Can you work these out from the drawing? Everything is in mm from the part's minimum corner. Coordinates: 2 decimals unless noted, no trailing zeros. Loops run counter-clockwise (first coordinate to the right, second up) from the corner with the lowest first, then second, coordinate; pieces in that order, holes last. Notation, with made-up numbers: (-14.5, 2.5) - (44.5, 2.5) arc R26 ccw to (44.5, 25.5) - close; hole circle Ø8 at (42, -11). An arc over 180 degrees is marked (long way). One line per question, with ' | ' between items. Start each with the question number.
1. I want a section at B-B, the plane y = 0.6. Count the separate pieces of the cut face and the enclosed holes in it, then the cut area to 3 significant figures.
2. I want a section at C-C, the plane z = 2.75. Write out the boundary of the cut face in (x, y).
3. I want a section at D-D, the plane x = 5.25. Write out the boundary of the cut face in (y, z), then the cut area to 3 significant figures.
4. We'd pull the mould along X, two halves only. Please class the marked faces 1, 2 and 3: pulls with the +X half, pulls with the -X half, needs draft (parallel to the pull), parting line crosses it, or undercut.
5. I'm going to push flat-ended pins straight in: P1, Ø1.3, axis at x = 7, y = 1.5, coming from the +Z side; P2, Ø1.3, axis at x = 10.5, y = 1, coming from the +Z side; P3, Ø0.6, axis at x = 7.5, y = 1, coming from the -Z side; P4, Ø4, axis at x = 14, z = 9.16, coming from the +Y side. Where does each tip first touch, or does it pass through?
6. I want a section at A-A, the plane x = 9. Write out the boundary of the cut face in (y, z).
7. Please list where these lines run through material, in increasing order: L1, parallel to X at y = 1, z = 9; L2, parallel to X at y = 1.55, z = 10.25; L3, parallel to X at y = 1.45, z = 11.25 (1 decimal). Write a range as [from, to].
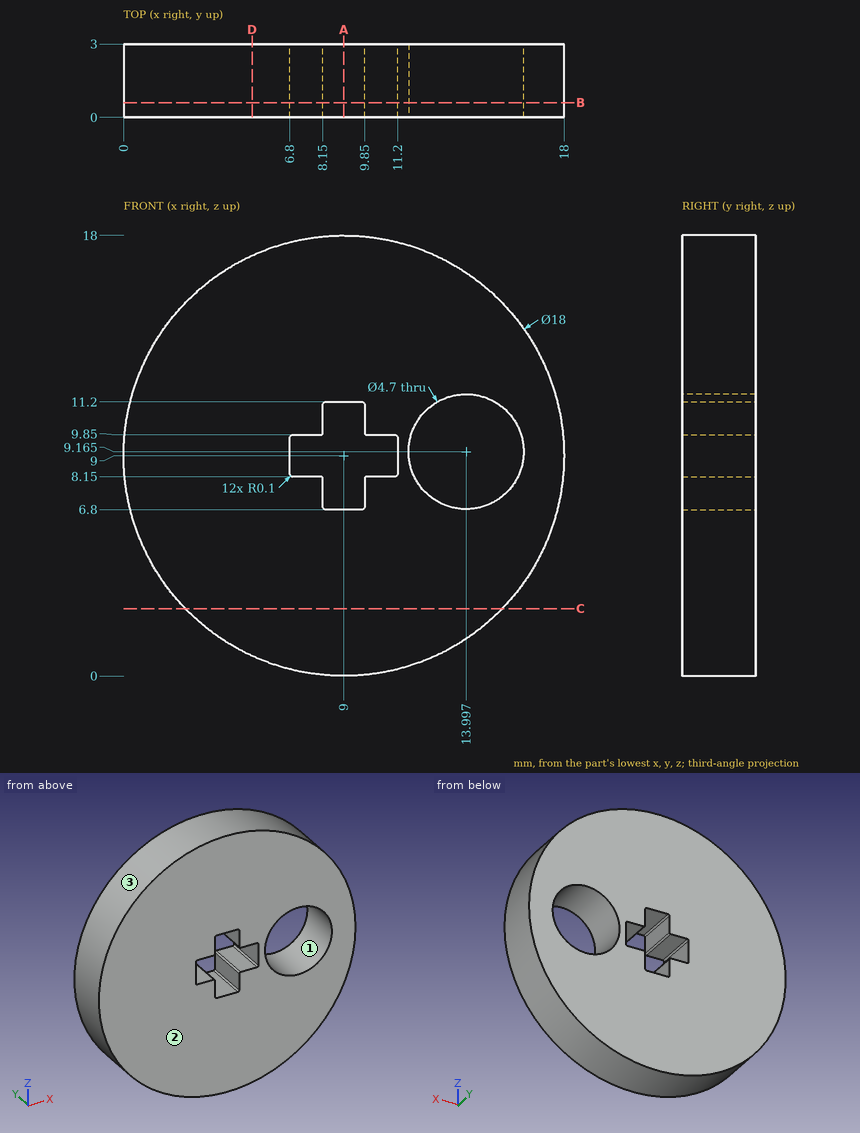
Results are:
1) separate pieces: 1 | enclosed holes: 2 | area: 225 mm2
2) outline: (2.52, 0) - (15.48, 0) - (15.48, 3) - (2.52, 3) - close
3) outline: (0, 0.82) - (3, 0.82) - (3, 17.18) - (0, 17.18) - close | area: 49.1 mm2
4) face 1: undercut | face 2: needs draft | face 3: parting line crosses it
5) P1: stops at z = 17.9 | P2: stops at z = 17.96 | P3: stops at z = 0.08 | P4: passes through
6) outline: (0, 0) - (3, 0) - (3, 6.8) - (0, 6.8) - close; (0, 11.2) - (3, 11.2) - (3, 18) - (0, 18) - close
7) L1: x = [0, 6.8], [11.2, 11.65], [16.34, 18] | L2: x = [0.09, 8.15], [9.85, 11.91], [16.08, 17.91] | L3: x = [0.3, 12.9], [15.1, 17.7]
